```python
from build123d import *

# Parameters (mm, degrees)
F0_R     = 11
F0_R_2   = 6
F1_DEPTH = 12
F2_SIZE  = 1
F3_R     = 2.625
F4_DEPTH = 12.5


with BuildPart() as f1:
    # F0 (on Front) → F1 (new body)
    with BuildSketch(Plane.XZ):
        Circle(F0_R)
        Circle(F0_R_2, mode=Mode.SUBTRACT)
    extrude(amount=-F1_DEPTH)

    # F2
    f2_edges = [f1.edges().sort_by_distance(p)[0] for p in [
        (-11, 12, 0),
    ]]
    chamfer(f2_edges, length=F2_SIZE)

    # F3 (on Right) → F4 (cut, symmetric)
    with BuildSketch(Plane.YZ):
        with Locations((6, 0)):
            Circle(F3_R)
    extrude(amount=F4_DEPTH, both=True, mode=Mode.SUBTRACT)


solid = f1.part
```
Can you work these out from the model? Positions are in its coordinate system, mm. Round coordinates to 2 decimals unless told otherwise and drop trailing zeros. Loops run counter-clockwise (first coordinate to the right, second up) from the corner with the lowest first, then second, coordinate; pieces in that order, holes last. Notation, with made-up numbers: (31, -17) -> (66, -17) arc R35 ccw to (66, 21) -> close; hole circle Ø7 at (37.5, -6.5). An arc over 180 degrees is marked (long way). One line per item, written item: value. Start each with the question number.
1. If we section it at C-C, the plane y = 2.25: Write out the boundary of the cut face in (x, z).
2. For pin 1 (3 mm diameter, centred on y = 6, z = -5, fed in from +X); pin 2 (5 mm diameter, centred on y = 2, z = -7.5, fed in from +X); pin 3 (1 mm diameter, centred on y = 8, z = -8.5, fed in from +X), each with a flat end and sliding along its axis, tell me the tip position at first contact or that it passes through.
3. If I drill on probe 1 along Z at (x, y) = (0, 5); probe 2 along Y at (x, z) = (7.05, 0) (3 decimals), over which ranges is the centre line in solid material (lowest first)?
4. If we section it at A-A, the plane x = 0: Write out the boundary of the cut face in (y, z), then the cut area to 3 significant figures.
5. If we mould it in two halves opening along Y, with no side actions, what happens to faces 1 (the flat face through (0, 12, -7)), 2 (the flat face through (5, 0, -5)), 3 (the cylindrical face through (8.237, 7.411, 2.213))? For each: pulls with the +Y half, pulls with the -Y half, needs draft (parallel to the pull), parting line crosses it, or undercut.
6. If we section it at D-D, the plane z = 2: Give the number of separate pieces and of enclosed holes in the cut face, then the cut area to 3 significant figures.
7. If we section it at B-B, the plane y = 4: Write out the boundary of the cut face in (x, z), then the cut area to 3 significant figures.
Calculated:
1. outline: circle Ø22 at (0, 0); hole circle Ø12 at (0, 0)
2. pin 1: stops at x = 10.43
2. pin 2: stops at x = 9.8
2. pin 3: stops at x = 7.55
3. probe 1: z = -11 to -6, 6 to 11
3. probe 2: y = 0 to 3.375, 8.625 to 12
4. outline: (0, -11) -> (11, -11) -> (12, -10) -> (12, -6) -> (0, -6) -> close; (0, 6) -> (12, 6) -> (12, 10) -> (11, 11) -> (0, 11) -> close
4. area: 119 mm²
5. face 1: pulls with the +Y half
5. face 2: pulls with the -Y half
5. face 3: undercut
6. separate pieces: 4
6. enclosed holes: 0
6. area: 87.7 mm²
7. outline: (-10.87, -1.7) arc R11 ccw to (10.87, -1.7) -> (5.75, -1.7) arc R6 cw to (-5.75, -1.7) -> close; (-10.87, 1.7) -> (-5.75, 1.7) arc R6 cw to (5.75, 1.7) -> (10.87, 1.7) arc R11 ccw to start
7. area: 233 mm²
